Job drawing, mm, ordinate dimensions from the low corner. One solid piece. A direction names the side the tool comes from. Round coordinates to 2 decimals unless told otherwise and drop trailing zeros. Loops run counter-clockwise (first coordinate to the right, second up) from the corner with the lowest first, then second, coordinate; pieces in that order, holes last. Notation, with made-up numbers: (29, 51.25) - (49, 51.25) arc R26 cw to (49, 73.25) - close; hole circle Ø2 at (68, 84). An arc over 180 degrees is marked (long way). One line per question, with ' | ' between items. Start each with the question number.
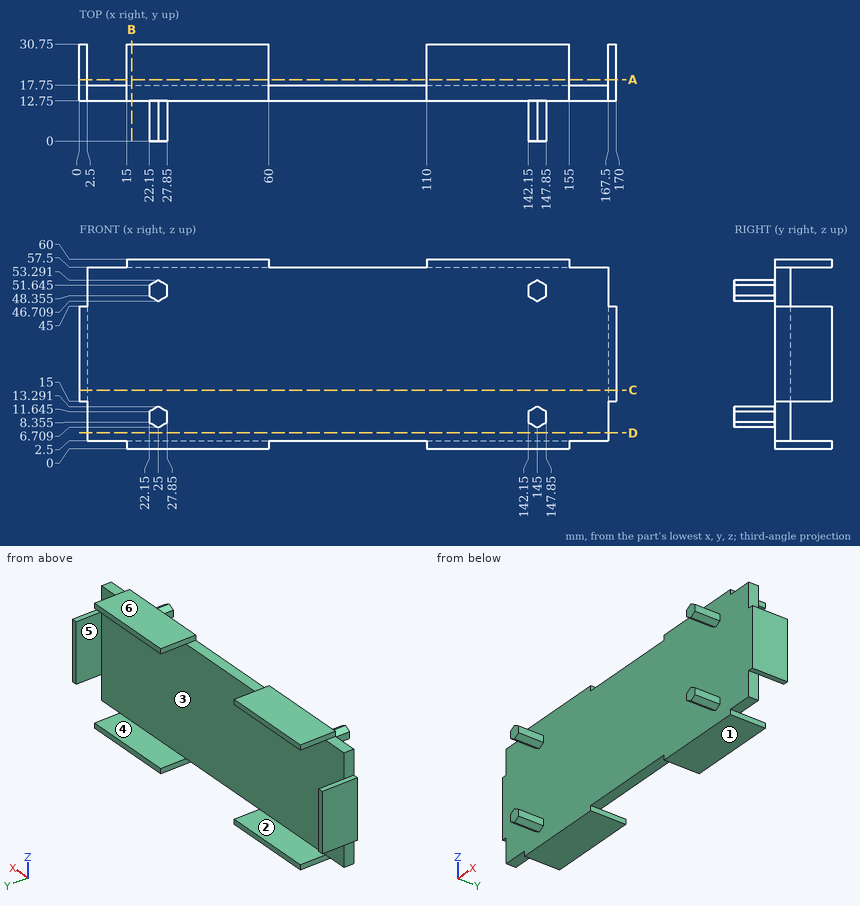
1) Saw through at A-A on y = 19.5. Write the cut outline in (x, z), and give its area (3 significant figures).
2) Wall check: line 1 (Z direction, x = 138.5, y = 27); line 2 (X direction, y = 21, z = 31.5); line 3 (Y direction, x = 54, z = 14). Give the ranges that are in metal, low to high. Write a range as [from, to].
3) Tool access for the marked faces 1, 2 and 3: list every direction of +Z, -Z, +X, -X, +Y, -Y with a clear straight run to the whole face (end or side of a thin tool).
4) Drop flat-ended pins along their axis: pin 1 (5.5 mm diameter, centred on x = 76.5, y = 16, fed in from +Z); pin 2 (3 mm diameter, centred on y = 25, z = 58.5, fed in from +X); pin 3 (18 mm diameter, centred on x = 75, z = 18.5, fed in from -Y). Give the stop position or say it passes through.
5) Two-plate mould, pull along Z, no slides. Class the marked faces 4, 5 and 6: +Z half, -Z half, draft (parallel to the pull), parting line (faces both ways), or undercut.
6) Saw through at B-B on x = 16.5. Write the cut outline in (y, z).
7) Saw through at D-D on z = 5. Write the cut outline in (x, y), and give its area (3 significant figures).
8) Saw through at C-C on z = 18.5. Write the cut outline in (x, y), and give its area (3 significant figures).
Answer key:
1) outline: (0, 15) - (2.5, 15) - (2.5, 45) - (0, 45) - close; (15, 0) - (60, 0) - (60, 2.5) - (15, 2.5) - close; (15, 57.5) - (60, 57.5) - (60, 60) - (15, 60) - close; (110, 0) - (155, 0) - (155, 2.5) - (110, 2.5) - close; (110, 57.5) - (155, 57.5) - (155, 60) - (110, 60) - close; (167.5, 15) - (170, 15) - (170, 45) - (167.5, 45) - close | area: 600 mm²
2) line 1: [0, 2.5], [57.5, 60] | line 2: [0, 2.5], [167.5, 170] | line 3: [12.75, 17.75]
3) face 1: -Z, +X, -X, +Y, -Y | face 2: +X, -X, +Y | face 3: +Y
4) pin 1: z = 57.5 | pin 2: x = 155 | pin 3: y = 12.75
5) face 4: undercut | face 5: draft | face 6: +Z half
6) outline: (12.75, 0) - (30.75, 0) - (30.75, 2.5) - (17.75, 2.5) - (17.75, 57.5) - (30.75, 57.5) - (30.75, 60) - (12.75, 60) - close
7) outline: (2.5, 12.75) - (167.5, 12.75) - (167.5, 17.75) - (2.5, 17.75) - close | area: 825 mm²
8) outline: (0, 12.75) - (170, 12.75) - (170, 30.75) - (167.5, 30.75) - (167.5, 17.75) - (2.5, 17.75) - (2.5, 30.75) - (0, 30.75) - close | area: 915 mm²
